Geometry check sheet. Reference: the model listing, model coordinates, mm. A direction names the side the tool comes from. Coordinates: 2 decimals unless noted, no trailing zeros. Order: outer loops, then holes, each group sorted by start corner. A loop starts at its lowest first (then second) coordinate and runs counter-clockwise, first axis right, second up. Notation, with made-up numbers: (30, 19) -> (40, 19) arc R17 ccw to (40, 51) -> close; hole circle Ø5 at (-2.75, 43.5). An arc over 180 degrees is marked (long way). Answer as CSV lines item,"result". Start each with the question number.
from build123d import *

# Parameters (mm, degrees)
SKETCH_1_R      = 21.5
EXTRUDE_1_DEPTH = 16
FILLET_1_R      = 8.5


with BuildPart() as part:
    # 草图1 → 凸台-拉伸1 (new body)
    with BuildSketch(Plane(origin=(0, 0, 0), x_dir=(1, 0, 0), z_dir=(0, 1, 0))):
        with Locations(Location((0, 0, 0), (0, 0, 270))):
            Circle(SKETCH_1_R)
        Polygon((9.526279442, -16.5), (19.052558883, 0), (9.526279442, 16.5), (-9.526279442, 16.5), (-19.052558883, 0), (-9.526279442, -16.5), align=None, mode=Mode.SUBTRACT)
    extrude(amount=EXTRUDE_1_DEPTH)

    # 圆角1
    fillet_1_edges = [part.edges().sort_by_distance(p)[0] for p in [
        (9.526279442, 8, 16.5),
        (19.052558883, 8, 0),
        (9.526279442, 8, -16.5),
        (-9.526279442, 8, -16.5),
        (-19.052558883, 8, 0),
        (-9.526279442, 8, 16.5),
    ]]
    fillet(fillet_1_edges, radius=FILLET_1_R)


solid = part.part
Q1. Access from +Z, -Z, +X, -X, +Y, -Y to the whole of each face (thin tool, end or side, straight path). Record for faces 1 (the flat face through (-14.257, 7.888, -8.306)), 2 (the flat face through (13, 0, 11)).
Q2. Thickness scan on L1, parallel to Z at x = 15, y = 7.5; L2, parallel to Z at x = -10.5, y = 11.75; L3, parallel to X at y = 14.5, z = -6. Record the ranges inside material, lowest first.
Q3. Sectioned sample at B-B, the plane z = 0. Record the cut outline in (x, y).
Q4. Go/stop test with flat-tipped pins: pin 1 Ø1.5 at (x, y) = (7.5, 7) entering from +Z; pin 2 Ø5 at (x, y) = (15.5, 13.5) entering from +Z; pin 3 Ø3 at (x, y) = (-1.5, 7.5) entering from -Z; pin 4 Ø2 at (x, y) = (11, 7.5) entering from +Z. Record where each tip stops, or that it passes through.
Q5. Sectioned sample at C-C, the plane y = 10.25. Record the cut outline in (x, z), then the cut area to 3 significant figures.
Q6. Sectioned sample at A-A, the plane x = 0. Record the cut outline in (y, z), then the cut area to 3 significant figures.
Q7. Release check for a two-part mould opening along X. For faces 3 (the cylindrical face through (14.531, 7.888, -15.846)), 4 (the flat face through (13, 16, 11)), 5 (the cylindrical face through (-17.737, 8.112, -0.062)) record: released by +X, released by -X, zero draft, split by the parting line, or undercut.
Geometry results:
1,face 1,"+Y, -Y"
1,face 2,"+Z, -Z, +X, -X, -Y"
2,L1,"z = -15.4 to -7.02, 7.02 to 15.4"
2,L2,"z = -18.76 to -14.14, 14.14 to 18.76"
2,L3,"x = -20.65 to -15.59, 15.59 to 20.65"
3,outline,"(-21.5, 0) -> (-17.74, 0) -> (-17.74, 16) -> (-21.5, 16) -> close; (17.74, 0) -> (21.5, 0) -> (21.5, 16) -> (17.74, 16) -> close"
4,pin 1,"stops at z = 20.41"
4,pin 2,"stops at z = 17.12"
4,pin 3,"stops at z = -21.5"
4,pin 4,"stops at z = 19.03"
5,outline,"circle Ø43 at (0, 0); hole (-16.6, -4.25) -> (-11.98, -12.25) arc R8.5 ccw to (-4.62, -16.5) -> (4.62, -16.5) arc R8.5 ccw to (11.98, -12.25) -> (16.6, -4.25) arc R8.5 ccw to (16.6, 4.25) -> (11.98, 12.25) arc R8.5 ccw to (4.62, 16.5) -> (-4.62, 16.5) arc R8.5 ccw to (-11.98, 12.25) -> (-16.6, 4.25) arc R8.5 ccw to start"
5,area,"532 mm^2"
6,outline,"(0, -21.5) -> (16, -21.5) -> (16, -16.5) -> (0, -16.5) -> close; (0, 16.5) -> (16, 16.5) -> (16, 21.5) -> (0, 21.5) -> close"
6,area,"160 mm^2"
7,face 3,"split by the parting line"
7,face 4,"zero draft"
7,face 5,"undercut"
